Could you check a few things on this model? Use its own coordinates, in mm. A direction names the side the tool comes from. Give positions to 0.01 mm unless a question says otherwise; leave off trailing zeros. One line per item, written item: value. Start each with the question number.
Q1. I'm going to push flat-ended pins straight in: P1, Ø2, axis at y = 4.5, z = 22.5, coming from the +X side; P2, Ø2, axis at y = 4.5, z = -22.5, coming from the -X side. Where does each tip first touch, or does it pass through?
Q2. For faces 4 (the face through (36.021, 4.979, -21.345)), 5 (the face through (37.5, 5, 0)), 6 (the face through (-36.021, 4.979, -21.345)), which set-ups out of +Z, -Z, +X, -X, +Y, -Y let a thin tool reach every point of the face, with its end or its side?
Q3. If we mould it in two halves opening along Y, with no side actions, what happens to faces 1 (the face through (-1, 9.5, 0)), 2 (the face through (33.88, 4.58, -22.3)), 3 (the face through (-32.82, 4.82, -21.29))? For each: released by +Y, released by -Y, zero draft, split by the parting line, or undercut.
Q4. If I drill on line 1 (Z direction, x = 35.65, y = 4.5); line 2 (X direction, y = 5.75, z = 21.5); line 3 (X direction, y = 5.5, z = -21), over which ranges is the centre line in solid material (lowest first)? Write a range as from..to.
```python
from build123d import *

# Parameters (mm, degrees)
SKETCH1_W                      = 75
SKETCH1_H                      = 55
BOSS_EXTRUDE1_DEPTH            = 9.5
SKETCH2_R                      = 1.35
CUT_EXTRUDE1_DEPTH             = 10
M3X0_5_TAPPED_HOLE2_AT_2_COUNT = 2
M3X0_5_TAPPED_HOLE2_AT_2_PITCH = 45


with BuildPart() as part:
    # Sketch1 → Boss-Extrude1 (new body)
    with BuildSketch(Plane(origin=(0, 0, 0), x_dir=(1, 0, 0), z_dir=(0, 1, 0))):
        Rectangle(SKETCH1_W, SKETCH1_H)
    extrude(amount=BOSS_EXTRUDE1_DEPTH)

    # Sketch2 → Cut-Extrude1 (cut)
    with BuildSketch(Plane(origin=(0, 9.5, 0), x_dir=(1, 0, 0), z_dir=(0, 1, 0))):
        with Locations(Location((-31.5, 21, 0), (0, 0, 270))):
            Circle(SKETCH2_R)
        with Locations(Location((31.420574921, 21.415697585, 0), (0, 0, 270))):
            Circle(SKETCH2_R)
        with Locations(Location((31.306542661, -21.346400068, 0), (0, 0, 270))):
            Circle(SKETCH2_R)
        with Locations(Location((-31.297168302, -20.548174245, 0), (0, 0, 270))):
            Circle(SKETCH2_R)
    extrude(amount=-CUT_EXTRUDE1_DEPTH, mode=Mode.SUBTRACT)

    # Sketch5 → M3x0.5 Tapped Hole2 (revolve, cut)
    with BuildSketch(Plane(origin=(-37.5, 4.5, -22.5), x_dir=(0, 0, 1), z_dir=(0, 1, 0))):
        Polygon((0, 0), (0, 3.751075774), (1.25, 3), (1.25, 0), align=None)
    m3x0_5_tapped_hole2 = revolve(axis=Axis((-43.85, 4.5, -22.5), (1, 0, 0)), mode=Mode.SUBTRACT)

    # M3x0.5 Tapped Hole2 at 2: M3x0.5 Tapped Hole2 ×2
    with Locations(*[(0, 0, i * M3X0_5_TAPPED_HOLE2_AT_2_PITCH) for i in range(1, M3X0_5_TAPPED_HOLE2_AT_2_COUNT)]):
        add(m3x0_5_tapped_hole2, mode=Mode.SUBTRACT)

    # Mirror1: M3x0.5 Tapped Hole2 across plane
    add(m3x0_5_tapped_hole2.mirror(Plane.ZY), mode=Mode.SUBTRACT)

    # Mirror1 copy 1 sketch → Mirror1 copy 1 (revolve, cut)
    with BuildSketch(Plane(origin=(37.5, 4.5, 22.5), x_dir=(0, 0, 1), z_dir=(0, 1, 0))):
        Polygon((0, 0), (0, -3.751075774), (1.25, -3), (1.25, 0), align=None)
    revolve(axis=Axis((43.85, 4.5, 22.5), (1, 0, 0)), mode=Mode.SUBTRACT)


solid = part.part
```
Worked answers:
1. P1: stops at x = 34.35
1. P2: stops at x = -34.35
2. face 4: +X
2. face 5: +Z, -Z, +X, +Y, -Y
2. face 6: -X
3. face 1: released by +Y
3. face 2: undercut
3. face 3: zero draft
4. line 1: z = -27.5..-23.75, -21.25..21.25, 23.75..27.5
4. line 2: x = -37.5..-32.25, -30.34..29.97, 32.65..37.5
4. line 3: x = -37.5..-32.85, -30.15..30.14, 32.7..37.5
